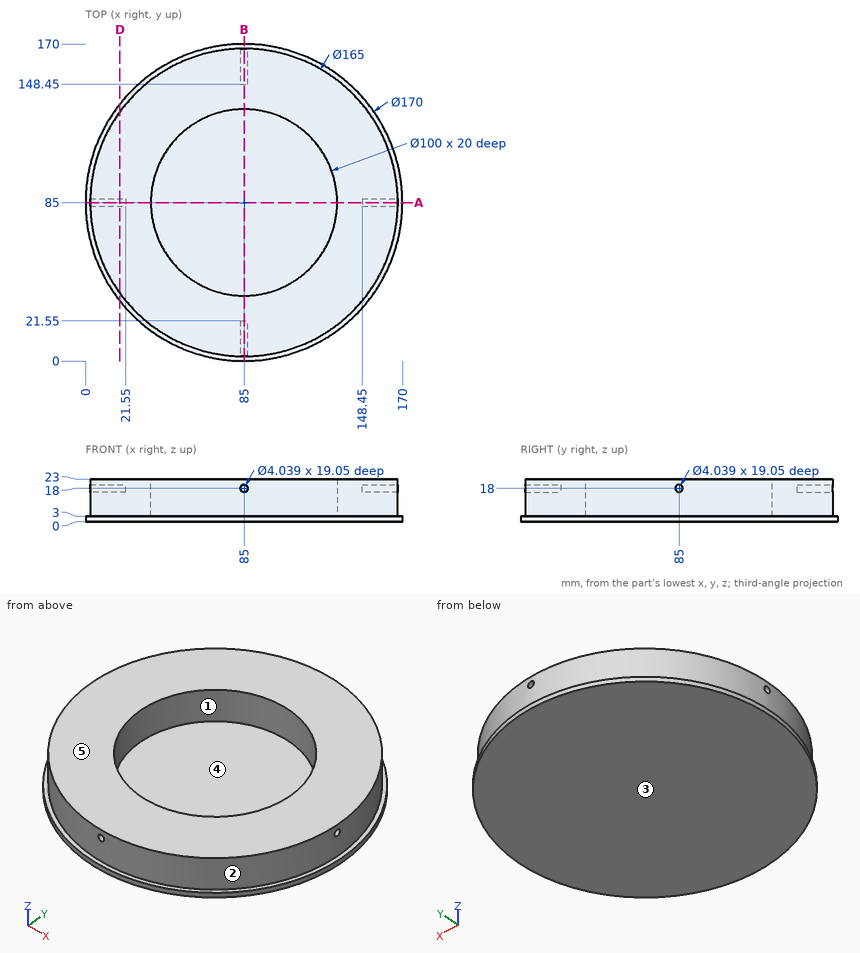
Geometry check sheet. Reference: drawing and pictorial views, mm from the part's lowest x, y, z. A direction names the side the tool comes from. Coordinates: 2 decimals unless noted, no trailing zeros. Order: outer loops, then holes, each group sorted by start corner. A loop starts at its lowest first (then second) coordinate and runs counter-clockwise, first axis right, second up. Notation, with made-up numbers: (63.5, 57) -> (95.5, 57) arc R20 cw to (95.5, 76) -> close; hole circle Ø3 at (-33.5, 30). An arc over 180 degrees is marked (long way). Put each result on its own line as item: value. Start each with the question number.
1) Material ranges on L1, parallel to Y at x = 85, z = 8.75; L2, parallel to Z at x = 54, y = 76; L3, parallel to Z at x = 85, y = 160.5, recorded low to high.
2) Cross-section at D-D (x = 18.5). Enter the section's corners in (y, z).
3) Cross-section at A-A (y = 85). Enter the section's corners in (x, z), plus the area to 3 significant figures.
4) Go/stop test with flat-tipped pins: pin 1 (4.5 mm diameter, centred on x = 85, z = 17.5, fed in from -Y); pin 2 (6 mm diameter, centred on x = 17.5, z = 7, fed in from -Y); pin 3 (2 mm diameter, centred on x = 85, z = 18.5, fed in from +Y). Record where each tip stops, or that it passes through.
5) Tool access check on the marked faces 4 and 5. Record the directions out of +Z, -Z, +X, -X, +Y, -Y that give a thin tool (end or side, any length) a straight path to the whole face; none if there is none.
6) Release check for a two-part mould opening along X. For the marked faces 1, 2 and 3 record: pulls with the +X half, pulls with the -X half, needs draft (parallel to the pull), parting line crosses it, or undercut.
Geometry check:
1. L1: y = 2.5 to 35, 135 to 167.5
1. L2: z = 0 to 3
1. L3: z = 0 to 15.98, 20.02 to 23
2. outline: (32.06, 0) -> (137.94, 0) -> (137.94, 3) -> (133.83, 3) -> (133.83, 23) -> (36.17, 23) -> (36.17, 3) -> (32.06, 3) -> close; hole circle Ø4.04 at (85, 18)
3. outline: (0, 0) -> (170, 0) -> (170, 3) -> (167.5, 3) -> (167.5, 15.98) -> (148.45, 15.98) -> (148.45, 20.02) -> (167.5, 20.02) -> (167.5, 23) -> (135, 23) -> (135, 3) -> (35, 3) -> (35, 23) -> (2.5, 23) -> (2.5, 20.02) -> (21.55, 20.02) -> (21.55, 15.98) -> (2.5, 15.98) -> (2.5, 3) -> (0, 3) -> close
3. area: 1,660 mm^2
4. pin 1: stops at y = 2.5
4. pin 2: stops at y = 33.56
4. pin 3: stops at y = 148.45
5. face 4: +Z
5. face 5: +Z, +X, -X, +Y, -Y
6. face 1: undercut
6. face 2: parting line crosses it
6. face 3: needs draft
